Read the model definition and answer for the solid it produces. Units are mm, in the model's axes. Give positions to 0.01 mm unless a question says otherwise; leave off trailing zeros. Order: outer loops, then holes, each group sorted by start corner. A loop starts at its lowest first (then second) coordinate and runs counter-clockwise, first axis right, second up.
Item 1: The mould has two halves that part along Y. Classify faces 1 (the face through (-40.4, -40.24, 1.01)), 2 (the face through (-43.25, 0, 1)), 3 (the face through (37.21, 35.88, 0.99)): +Y half, -Y half, draft (parallel to the pull), parting line (faces both ways), or undercut.
Item 2: Given pin 1 Ø4 at (x, y) = (-35.5, -35.5) entering from +Z, flat-ended and moving along its own axis, determine where the tip first touches the part or whether it passes through.
Item 3: A cutting plane is placed at A-A (z = 1.6). Write down the section's boundary in (x, y), plus the area to 3 significant figures.
Item 4: Find the intervals of material crossed by line 1 along X through (y, z) = (35.5, 1.55); line 2 along Y through (x, z) = (37, 0.5); line 3 along X through (y, z) = (-36, 0.4), in increasing order.
Item 5: A cutting plane is placed at B-B (y = 35.5). Write down the section's boundary in (x, z), plus the area to 3 significant figures.
Autodesk Fusion 360 part; units mm, degrees
sketch "Sketch1" plane through (0, 0, 0) normal (0, 0, 1) x (1, 0, 0)
  line L0 (43.25, 43.25) -> (-43.25, 43.25)
  line L1 (-43.25, 43.25) -> (-43.25, -43.25)
  line L2 (-43.25, -43.25) -> (43.25, -43.25)
  line L3 (43.25, -43.25) -> (43.25, 43.25)
  line L4 (43.25, 43.25) -> (-43.25, -43.25) construction
  line L5 (-43.25, 43.25) -> (43.25, -43.25) construction
  dimension "d17" = 86.5
  dimension "d18" = 86.5
extrude "Extrude1" add sketch "Sketch1" along normal blind 2
fillet "Fillet1" radius 10 1 edges at (-43.25, -43.25, 1)
fillet "Fillet2" radius 10 1 edges at (43.25, -43.25, 1)
fillet "Fillet3" radius 10 1 edges at (43.25, 43.25, 1)
fillet "Fillet4" radius 10 1 edges at (-43.25, 43.25, 1)
sketch "Sketch2" plane through (0, 0, 2) normal (0, 0, 1) x (-1, 0, 0)
  arc A0 (33.25, -43.25) -> (43.25, -33.25) centre (33.25, -33.25) ccw
  line L0 (43.25, -33.25) -> (43.25, 33.25)
  arc A1 (43.25, 33.25) -> (33.25, 43.25) centre (33.25, 33.25) ccw
  line L1 (33.25, 43.25) -> (-33.25, 43.25)
  arc A2 (-33.25, 43.25) -> (-43.25, 33.25) centre (-33.25, 33.25) ccw
  line L2 (-43.25, 33.25) -> (-43.25, -33.25)
  arc A3 (-43.25, -33.25) -> (-33.25, -43.25) centre (-33.25, -33.25) ccw
  line L3 (-33.25, -43.25) -> (33.25, -43.25)
  point P0 (35.5, -35.5)
  point P1 (-35.5, -35.5)
  point P2 (-35.5, 35.5)
  point P3 (35.5, 35.5)
  dimension "d25" = 35.5
  dimension "d26" = 35.5
  dimension "d27" = 71
  dimension "d28" = 71
hole "Hole1" at (-35.5, 35.5, 2) at (35.5, 35.5, 2) at (35.5, -35.5, 2) at (-35.5, -35.5, 2) direction (0, 0, -1) diameter 3.5 depth 30 tip angle 118
Response values:
1. face 1: -Y half
1. face 2: draft
1. face 3: undercut
2. pin 1: stops at z = 2
3. outline: (-43.25, -33.25) arc R10 ccw to (-33.25, -43.25) - (33.25, -43.25) arc R10 ccw to (43.25, -33.25) - (43.25, 33.25) arc R10 ccw to (33.25, 43.25) - (-33.25, 43.25) arc R10 ccw to (-43.25, 33.25) - close; hole circle Ø3.5 at (-35.5, -35.5); hole circle Ø3.5 at (-35.5, 35.5); hole circle Ø3.5 at (35.5, -35.5); hole circle Ø3.5 at (35.5, 35.5)
3. area: 7,360 mm2
4. line 1: x = -42.99 to -37.25, -33.75 to 33.75, 37.25 to 42.99
4. line 2: y = -42.52 to -36.4, -34.6 to 34.6, 36.4 to 42.52
4. line 3: x = -42.86 to -37.18, -33.82 to 33.82, 37.18 to 42.86
5. outline: (-42.99, 0) - (-37.25, 0) - (-37.25, 2) - (-42.99, 2) - close; (-33.75, 0) - (33.75, 0) - (33.75, 2) - (-33.75, 2) - close; (37.25, 0) - (42.99, 0) - (42.99, 2) - (37.25, 2) - close
5. area: 158 mm2
